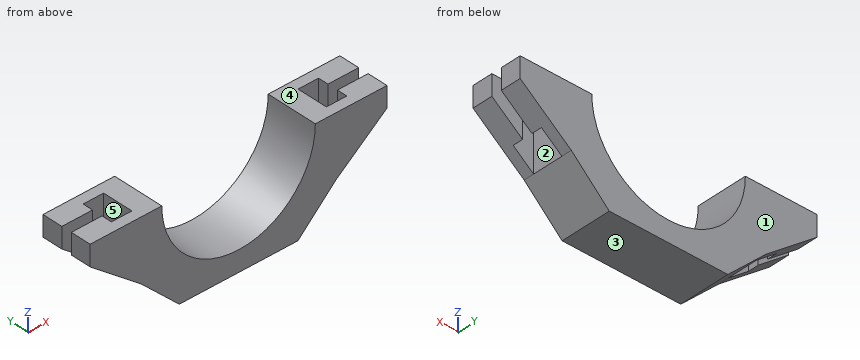
```python
from build123d import *

# Parameters (mm, degrees)
F0_W      = 5
F0_H      = 2
F1_DEPTH  = 2.5
F5_DEPTH  = 5
F6_W      = 3
F6_H      = 1
F6_W_2    = 2
F7_DEPTH  = 25
F8_DEPTH  = 25
F9_DEPTH  = 19
F11_DEPTH = 25


with BuildPart() as f1:
    # F0 (on Front) → F1 (new body, symmetric)
    with BuildSketch(Plane.XZ):
        with BuildLine():
            ThreePointArc((6.25, 0), (-1.25, -7.5), (-8.75, 0))
            Line((-8.75, 0), (-10.75, 0))
            ThreePointArc((-10.75, 0), (-7.9675144213, -6.7175144213), (-1.25, -9.5))
            ThreePointArc((-1.25, -9.5), (5.4675144213, -6.7175144213), (8.25, 0))
            Line((8.25, 0), (6.25, 0))
        make_face()
        with BuildLine():
            ThreePointArc((-1.25, -9.5), (-7.9675144213, -6.7175144213), (-10.75, 0))
            Line((-10.75, 0), (-10.75, -2))
            Line((-10.75, -2), (-10.75, -9.5))
            Line((-10.75, -9.5), (-1.25, -9.5))
        make_face()
        with Locations((-13.25, -1)):
            Rectangle(F0_W, F0_H)
        with BuildLine():
            Line((8.25, -2), (8.25, 0))
            ThreePointArc((8.25, 0), (5.4675144213, -6.7175144213), (-1.25, -9.5))
            Line((-1.25, -9.5), (8.25, -9.5))
            Line((8.25, -9.5), (8.25, -2))
        make_face()
        with Locations((10.75, -1)):
            Rectangle(F0_W, F0_H)
    extrude(amount=F1_DEPTH, both=True)

    # F4 (on face) → F5 (join, through all)
    with BuildSketch(Plane.XZ.offset(2.5)):
        Polygon((-10.75, -2), (-15.75, -2), (-10.75, -5.9285714286), align=None)
        Polygon((8.25, -5.9285714286), (13.25, -2), (8.25, -2), align=None)
    extrude(amount=-F5_DEPTH)

    # F6 (on face) → F7 (cut)
    with BuildSketch(Plane.XY):
        with Locations((-14.25, 0)):
            Rectangle(F6_W, F6_H)
        with Locations((-11.75, 1)):
            Rectangle(F6_W_2, F6_H)
        with Locations((-11.75, 0)):
            Rectangle(F6_W_2, F6_H)
        with Locations((-11.75, -1)):
            Rectangle(F6_W_2, F6_H)
        Polygon((13.25, -0.500000013), (13.25, 0.499999987), (10.2499989308, 0.499999987), (10.2499989308, 1.499999987), (8.2499989308, 1.499999987), (8.2499989308, -1.500000013), (10.2499989308, -1.500000013), (10.2499989308, -0.500000013), align=None)
    extrude(amount=-F7_DEPTH, mode=Mode.SUBTRACT)

    # F3 (on face) → F8 (cut)
    with BuildSketch(Plane.YZ.offset(8.25)):
        Polygon((2.5, -9.5), (2.5, -8.1602540378), (-2.5, -9.5), align=None)
    extrude(amount=-F8_DEPTH, mode=Mode.SUBTRACT)

    # F3 (on face) → F9 (join, through all)
    with BuildSketch(Plane.YZ.offset(8.25)):
        Polygon((2.5, -9.5), (2.5, -8.1602540378), (-2.5, -9.5), align=None)
    extrude(amount=-F9_DEPTH)

    # F10 (on face) → F11 (cut)
    with BuildSketch(Plane.XZ.offset(2.5)):
        Polygon((-10.75, -9.5), (-7.04318, -9.5), (-10.75, -5.9285714286), align=None)
        Polygon((8.25, -5.9285714286), (4.54318, -9.5), (8.25, -9.5), align=None)
    extrude(amount=-F11_DEPTH, mode=Mode.SUBTRACT)


solid = f1.part
```
Check sheet for the modelled part. Datum: model origin and axes. Units: mm. Face numbers are marked on the shaded views. A direction names the side the tool comes from. Give positions to 0.01 mm unless a question says otherwise; leave off trailing zeros. Order: outer loops, then holes, each group sorted by start corner. A loop starts at its lowest first (then second) coordinate and runs counter-clockwise, first axis right, second up. Notation, with made-up numbers: M 16.5,83.25 L 55.5,83.25 A25 cw 55.5,109.25 Z; hole C -2.75,-1.75 d6. An arc over 180 degrees is marked long. Answer in a Markdown table with one row per item.
1) Cross-section at A-A, the plane y = -1.2. Enter the section's corners in (x, z), plus the area to 3 significant figures.
Filled sheet:
| item | result |
|---|---|
| outline | M -15.75,-2 L -12.75,-4.36 L -12.75,0 L -15.75,0 Z; M -10.75,-5.93 L -7.04,-9.5 L 4.54,-9.5 L 8.25,-5.93 L 8.25,0 L 6.25,0 A7.5 cw -8.75,0 L -10.75,0 Z; M 10.25,-4.36 L 13.25,-2 L 13.25,0 L 10.25,0 Z |
| area | 98.0 mm2 |
2) Release check for a two-part mould opening along Y. For the marked faces 1, 2 and 3 record: +Y half, -Y half, draft (parallel to the pull), parting line (faces both ways), or undercut.
Filled sheet:
| item | result |
|---|---|
| face 1 | +Y half |
| face 2 | undercut |
| face 3 | draft |
3) Cross-section at C-C, the plane z = -3.75. Enter the section's corners in (x, y), plus the area to 3 significant figures.
Filled sheet:
| item | result |
|---|---|
| outline | M -13.52,-2.5 L -7.75,-2.5 L -7.75,2.5 L -13.52,2.5 L -13.52,0.5 L -12.75,0.5 L -12.75,1.5 L -10.75,1.5 L -10.75,-1.5 L -12.75,-1.5 L -12.75,-0.5 L -13.52,-0.5 Z; M 5.25,-2.5 L 11.02,-2.5 L 11.02,-0.5 L 10.25,-0.5 L 10.25,-1.5 L 8.25,-1.5 L 8.25,1.5 L 10.25,1.5 L 10.25,0.5 L 11.02,0.5 L 11.02,2.5 L 5.25,2.5 Z |
| area | 44.2 mm2 |
4) Cross-section at B-B, the plane x = -11.5. Enter the section's corners in (y, z).
Filled sheet:
| item | result |
|---|---|
| outline | M -2.5,-5.34 L -1.5,-5.34 L -1.5,0 L -2.5,0 Z; M 1.5,-5.34 L 2.5,-5.34 L 2.5,0 L 1.5,0 Z |
5) Thickness scan on L1, parallel to X at y = 1.45, z = -0.25; L2, parallel to Y at x = 8.5, z = -1; L3, parallel to X at y = -1.4, z = -1.5. Record the ranges inside material, lowest first. Write a range as [from, to].
Filled sheet:
| item | result |
|---|---|
| L1 | x = [-15.75, -12.75], [-10.75, -8.75], [6.25, 8.25], [10.25, 13.25] |
| L2 | y = [-2.5, -1.5], [1.5, 2.5] |
| L3 | x = [-15.75, -12.75], [-10.75, -8.6], [6.1, 8.25], [10.25, 13.25] |
6) Cross-section at D-D, the plane y = 0.05. Enter the section's corners in (x, z).
Filled sheet:
| item | result |
|---|---|
| outline | M -10.75,-5.93 L -7.04,-9.5 L 4.54,-9.5 L 8.25,-5.93 L 8.25,0 L 6.25,0 A7.5 cw -8.75,0 L -10.75,0 Z |
7) Access from +Z, -Z, +X, -X, +Y, -Y to the whole of each face (thin tool, end or side, straight path). Record for the marked faces 4 and 5.
Filled sheet:
| item | result |
|---|---|
| face 4 | +Z, +X, -X, +Y, -Y |
| face 5 | +Z, -Z |
8) Gauge pin test, flat ends, axial feed: P1, Ø1.5, axis at y = 0, z = -4.5, coming from the -X side; P2, Ø3, axis at y = 2, z = -7, coming from the +X side; P3, Ø1.5, axis at y = 0.5, z = -6.5, coming from the +X side. Record the tip position at first contact, or that the pin passes through.
Filled sheet:
| item | result |
|---|---|
| P1 | stops at x = -13.28 |
| P2 | stops at x = 8.8 |
| P3 | stops at x = 8.25 |
